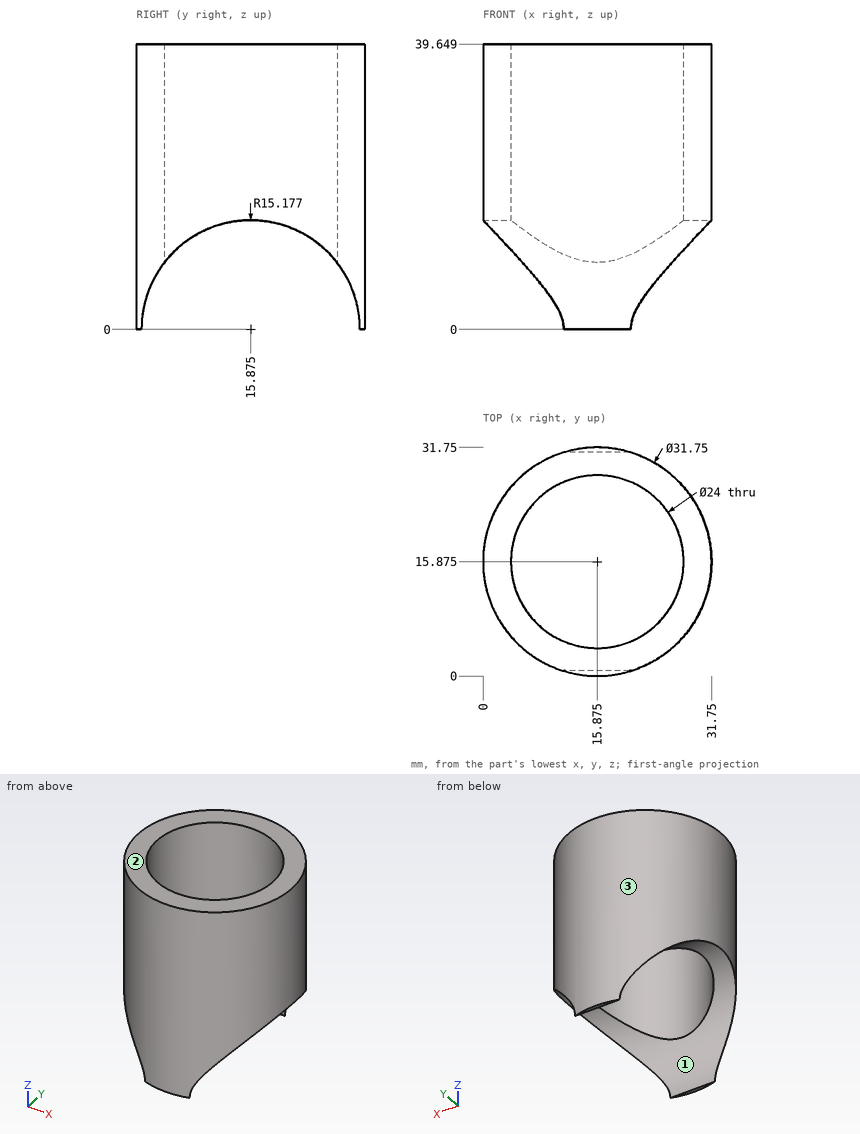
Job drawing, mm, ordinate dimensions from the low corner. One solid piece. Give positions to 0.01 mm unless a question says otherwise; leave off trailing zeros. Put each result on its own line as item: value. Start each with the question number.
(1) Drill centre lines: L1, parallel to Y at x = 24, z = 19.5 (1 decimal); L2, parallel to X at y = 12, z = 35; L3, parallel to Y at x = 23.5, z = 13. Where is each one in solid material? Low to high. Write a range as [from, to].
(2) Pull direction Y, two halves, no side cores. Call the marked faces 1, 2 and 3: released by +Y, released by -Y, zero draft, split by the parting line, or undercut.
(3) Pin check, flat tips, straight feed: pin 1 Ø6 at (x, z) = (6.5, 26) entering from +Y; pin 2 Ø1.5 at (y, z) = (23.5, 23) entering from -X (1 decimal); pin 3 Ø3 at (x, z) = (12, 7.5) entering from +Y; pin 4 Ø4 at (x, y) = (8.5, 9) entering from +Z. Stop position of each tip, or through.
Results below:
1. L1: y = [2.2, 7], [24.7, 29.5]
1. L2: x = [0.48, 4.52], [27.23, 31.27]
1. L3: y = [1.95, 6.61], [25.14, 29.8]
2. face 1: undercut
2. face 2: zero draft
2. face 3: split by the parting line
3. pin 1: stops at y = 30.41
3. pin 2: stops at x = 1.6
3. pin 3: stops at y = 31.57
3. pin 4: stops at z = 39.65
